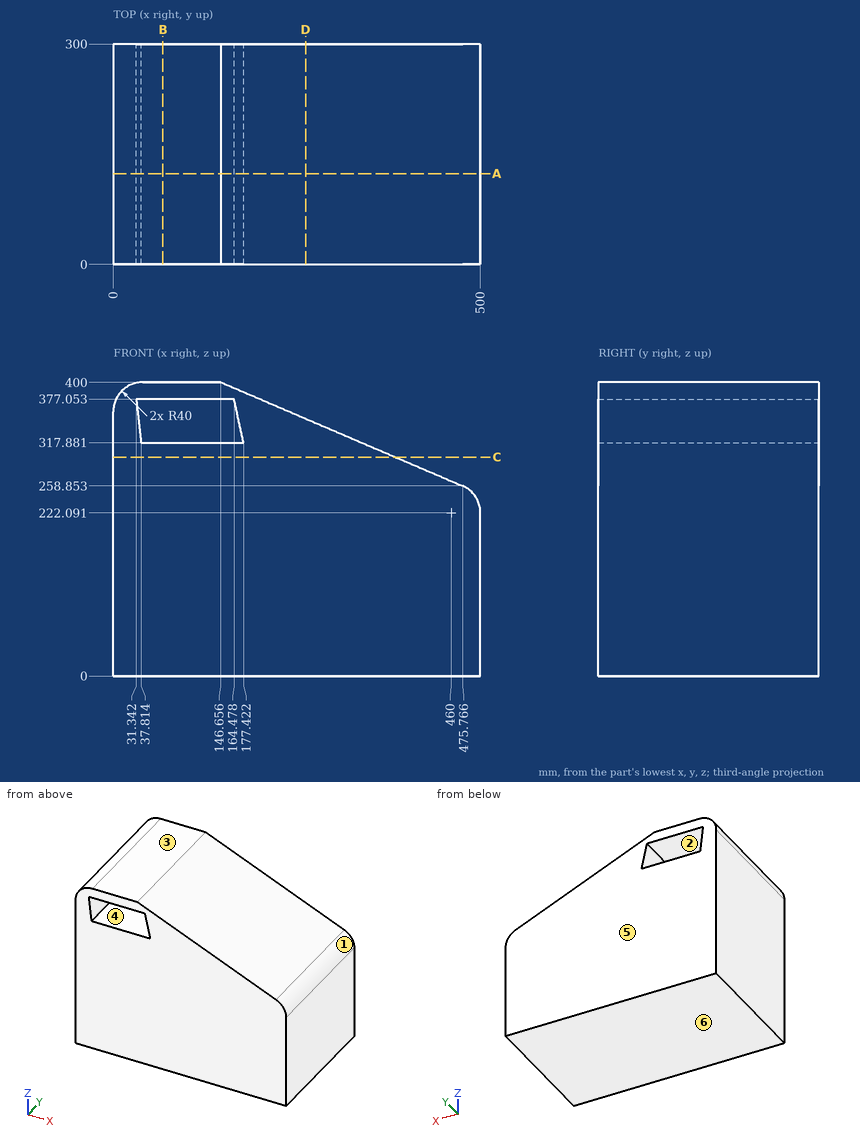
Geometry check sheet. Reference: drawing and pictorial views, mm from the part's lowest x, y, z. A direction names the side the tool comes from. Round coordinates to 2 decimals unless told otherwise and drop trailing zeros. Loops run counter-clockwise (first coordinate to the right, second up) from the corner with the lowest first, then second, coordinate; pieces in that order, holes last. Notation, with made-up numbers: (-18.75, 89.5) -> (6.25, 89.5) arc R10 cw to (6.25, 95.5) -> close; hole circle Ø2 at (36.25, 5.25). An arc over 180 degrees is marked (long way). Answer as a JSON object with one key per item and string values. Group by question number.
Item 1: Cross-section at A-A, the plane y = 123.5. Record the cut outline in (x, z) (1 decimal), plus the area to 3 significant figures.
Item 2: Cross-section at B-B, the plane x = 67.5. Record the cut outline in (y, z), plus the area to 3 significant figures.
Item 3: Set-up check for the marked faces 1 and 2: record each of +Z, -Z, +X, -X, +Y, -Y from which the full face is reachable in a straight line by a thin tool's end or side.
Item 4: Cross-section at D-D, the plane x = 262. Record the cut outline in (y, z), plus the area to 3 significant figures.
Item 5: Thickness scan on line 1 along Z through (x, y) = (59, 111); line 2 along X through (y, z) = (42, 332) (1 decimal); line 3 along Z through (x, y) = (164, 194.5). Record the ranges inside material, lowest first.
Item 6: Depth check by flat-ended pin: pin 1 Ø5 at (x, z) = (60, 179) entering from -Y; pin 2 Ø10 at (y, z) = (168, 284) entering from +X. Enter the tip coordinate at first touch or a pass-through.
Item 7: Cross-section at C-C, the plane z = 298. Record the cut outline in (x, y).
Item 8: Release check for a two-part mould opening along Z. For the marked faces 3, 4, 5 and 6 record: pulls with the +Z half, pulls with the -Z half, needs draft (parallel to the pull), parting line crosses it, or undercut.
Determined:
{
 "1": {"outline": "(0, 0) -> (500, 0) -> (500, 222.1) arc R40 ccw to (475.8, 258.9) -> (146.7, 400) -> (40, 400) arc R40 ccw to (0, 360) -> close; hole (31.3, 377.1) -> (37.8, 317.9) -> (177.4, 317.9) -> (164.5, 377.1) -> close", "area": "165,000 mm²"},
 "2": {"outline": "(0, 0) -> (300, 0) -> (300, 317.88) -> (0, 317.88) -> close; (0, 377.05) -> (300, 377.05) -> (300, 400) -> (0, 400) -> close", "area": "102,000 mm²"},
 "3": {"face 1": "+Z, +X, +Y, -Y", "face 2": "+Y, -Y"},
 "4": {"outline": "(0, 0) -> (300, 0) -> (300, 350.53) -> (0, 350.53) -> close", "area": "105,000 mm²"},
 "5": {"line 1": "z = 0 to 317.88, 377.05 to 400", "line 2": "x = 0 to 36.3, 174.3 to 305.2", "line 3": "z = 0 to 317.88, 377.05 to 392.56"},
 "6": {"pin 1": "stops at y = 0", "pin 2": "stops at x = 428.79"},
 "7": {"outline": "(0, 0) -> (384.49, 0) -> (384.49, 300) -> (0, 300) -> close"},
 "8": {"face 3": "pulls with the +Z half", "face 4": "undercut", "face 5": "needs draft", "face 6": "pulls with the -Z half"}
}
